Source: CAD feature listing. Evaluate the final solid. Frame: model axes, mm. A direction names the side the tool comes from. Coordinates: 2 decimals unless noted, no trailing zeros. Write each loop counter-clockwise with the first axis right and the second up, starting at its lowest first coordinate (ties: lowest second). Pieces come first, ordered by that corner, then holes. Notation, with made-up numbers: (36, 85) -> (90, 85) arc R9 cw to (90, 93) -> close; hole circle Ø6 at (48.5, -28). An arc over 180 degrees is marked (long way). Write item = value, one per line.
from build123d import *

# Parameters (mm, degrees)
SKIZZE1_R                       = 18.5
AUFSATZ_LINEAR_AUSTRAGEN1_DEPTH = 2
SKIZZE2_R                       = 17.5
AUFSATZ_LINEAR_AUSTRAGEN2_DEPTH = 7.2
SKIZZE3_R                       = 18.5
AUFSATZ_LINEAR_AUSTRAGEN3_DEPTH = 2
SKIZZE4_R                       = 10
AUFSATZ_LINEAR_AUSTRAGEN4_DEPTH = 6.8
SKIZZE5_R                       = 2.5
SCHNITT_LINEAR_AUSTRAGEN1_DEPTH = 32.756889016


with BuildPart() as part:
    # Skizze1 → Aufsatz-Linear austragen1 (new body)
    with BuildSketch(Plane(origin=(0, 0, 0), x_dir=(1, 0, 0), z_dir=(0, 1, 0))):
        with Locations(Location((0, 0, 0), (0, 0, 270))):
            Circle(SKIZZE1_R)
    extrude(amount=AUFSATZ_LINEAR_AUSTRAGEN1_DEPTH)

    # Skizze2 → Aufsatz-Linear austragen2 (add)
    with BuildSketch(Plane(origin=(0, 2, 0), x_dir=(1, 0, 0), z_dir=(0, 1, 0))):
        with Locations(Location((0, 0, 0), (0, 0, 270))):
            Circle(SKIZZE2_R)
    extrude(amount=AUFSATZ_LINEAR_AUSTRAGEN2_DEPTH)

    # Skizze3 → Aufsatz-Linear austragen3 (add)
    with BuildSketch(Plane(origin=(0, 9.2, 0), x_dir=(1, 0, 0), z_dir=(0, 1, 0))):
        with Locations(Location((0, 0, 0), (0, 0, 270))):
            Circle(SKIZZE3_R)
    extrude(amount=AUFSATZ_LINEAR_AUSTRAGEN3_DEPTH)

    # Skizze4 → Aufsatz-Linear austragen4 (add)
    with BuildSketch(Plane(origin=(0, 11.2, 0), x_dir=(1, 0, 0), z_dir=(0, 1, 0))):
        with Locations(Location((0, 0, 0), (0, 0, 270))):
            Circle(SKIZZE4_R)
    extrude(amount=AUFSATZ_LINEAR_AUSTRAGEN4_DEPTH)

    # Skizze5 → Schnitt-Linear austragen1 (cut, through all)
    with BuildSketch(Plane(origin=(0, 18, 0), x_dir=(1, 0, 0), z_dir=(0, 1, 0))):
        with Locations(Location((0, 0, 0), (0, 0, 270))):
            Circle(SKIZZE5_R)
    extrude(amount=-SCHNITT_LINEAR_AUSTRAGEN1_DEPTH, mode=Mode.SUBTRACT)


solid = part.part
1) Cut plane A-A, the plane z = 0. Output: boundary loops of the cut face in (x, y), and give its area (3 significant figures).
Answer block:
outline = (-18.5, 0) -> (-2.5, 0) -> (-2.5, 18) -> (-10, 18) -> (-10, 11.2) -> (-18.5, 11.2) -> (-18.5, 9.2) -> (-17.5, 9.2) -> (-17.5, 2) -> (-18.5, 2) -> close; (2.5, 0) -> (18.5, 0) -> (18.5, 2) -> (17.5, 2) -> (17.5, 9.2) -> (18.5, 9.2) -> (18.5, 11.2) -> (10, 11.2) -> (10, 18) -> (2.5, 18) -> close
area = 446 mm2
2) Cut plane D-D, the plane x = 11. Output: boundary loops of the cut face in (y, z), and give its area (3 significant figures).
Answer block:
outline = (0, -14.87) -> (2, -14.87) -> (2, -13.61) -> (9.2, -13.61) -> (9.2, -14.87) -> (11.2, -14.87) -> (11.2, 14.87) -> (9.2, 14.87) -> (9.2, 13.61) -> (2, 13.61) -> (2, 14.87) -> (0, 14.87) -> close
area = 315 mm2
3) Pull-direction query (Z, two-part tool) for faces 4 (the cylindrical face through (-10.648, 5.55, -13.887)), 5 (the flat face through (-2, 18, 2)), 6 (the cylindrical face through (-2.44, 9.13, -0.54)); classes: +Z half, -Z half, draft (parallel to the pull), parting line (faces both ways), or undercut.
Answer block:
face_4 = parting line
face_5 = draft
face_6 = undercut
4) Cut plane B-B, the plane x = 0. Output: boundary loops of the cut face in (y, z).
Answer block:
outline = (0, -18.5) -> (2, -18.5) -> (2, -17.5) -> (9.2, -17.5) -> (9.2, -18.5) -> (11.2, -18.5) -> (11.2, -10) -> (18, -10) -> (18, -2.5) -> (0, -2.5) -> close; (0, 2.5) -> (18, 2.5) -> (18, 10) -> (11.2, 10) -> (11.2, 18.5) -> (9.2, 18.5) -> (9.2, 17.5) -> (2, 17.5) -> (2, 18.5) -> (0, 18.5) -> close
5) First-contact query: pin 1 Ø6 at (x, y) = (-5.5, 15) entering from +Z; pin 2 Ø2 at (x, z) = (-12.5, 7) entering from +Y; pin 3 Ø3 at (y, z) = (13, -1) entering from -X. Flat tips, straight axial feed; report the tip coordinate or a pass-through.
Answer block:
pin_1 = 9.68
pin_2 = 11.2
pin_3 = -10
6) Cut plane C-C, the plane y = 15.5. Output: boundary loops of the cut face in (x, z), and give its area (3 significant figures).
Answer block:
outline = circle Ø20 at (0, 0); hole circle Ø5 at (0, 0)
area = 295 mm2
7) Material intervals for probe 1 along X at (y, z) = (12.25, 0); probe 2 along X at (y, z) = (6, 0); probe 3 along Y at (x, z) = (-12, 9.5), sorted ascending. Write a range as [from, to].
Answer block:
probe_1 = [-10, -2.5], [2.5, 10]
probe_2 = [-17.5, -2.5], [2.5, 17.5]
probe_3 = [0, 11.2]
8) Reachability of faces 1 (the cylindrical face through (-7.086, 10.186, 17.089)), 2 (the flat face through (-14, 9.2, -11)), 3 (the flat face through (-8, 11.2, 8)) from +Z, -Z, +X, -X, +Y, -Y: full face, straight path, thin tool, end or side. Return the list, or none.
Answer block:
face_1 = +Y, -Y
face_2 = none
face_3 = +Y
